from build123d import *

# Parameters (mm, degrees)
BOSS_EXTRUDE1_DEPTH = 3.175
CUT_EXTRUDE1_DEPTH  = 10
SKETCH3_R           = 2.0193
BOSS_EXTRUDE2_DEPTH = 3.175
FILLET1_R           = 10
FILLET2_R           = 50
SKETCH4_R           = 2.02
CUT_EXTRUDE2_DEPTH  = 10
SKETCH5_R           = 2.0193
BOSS_EXTRUDE3_DEPTH = 3.175
SKETCH6_W           = 3.175
SKETCH6_H           = 346.1216
CUT_EXTRUDE3_DEPTH  = 131.549169731


with BuildPart() as part:
    # Sketch1 → Boss-Extrude1 (new body)
    with BuildSketch(Plane.XY):
        Polygon((165.934536959, -16.66935), (157.315236959, -8.05005), (115.359952094, -8.05005), (89.959952094, -8.05005), (48.004667228, -8.05005), (39.385367228, -16.66935), (39.385367228, -40.05005), (39.385367228, -52.41105), (165.934536959, -56.67505), (165.934536959, -42.05005), align=None)
        with BuildLine():
            ThreePointArc((47.685367228, -44.38075), (49.704667228, -46.40005), (47.685367228, -48.41935))
            ThreePointArc((47.685367228, -48.41935), (45.666067228, -46.40005), (47.685367228, -44.38075))
        make_face(mode=Mode.SUBTRACT)
        with BuildLine():
            ThreePointArc((47.685367228, -12.63075), (49.704667228, -14.65005), (47.685367228, -16.66935))
            ThreePointArc((47.685367228, -16.66935), (45.666067228, -14.65005), (47.685367228, -12.63075))
        make_face(mode=Mode.SUBTRACT)
        with BuildLine():
            ThreePointArc((73.085367228, -44.38075), (75.104667228, -46.40005), (73.085367228, -48.41935))
            ThreePointArc((73.085367228, -48.41935), (71.066067228, -46.40005), (73.085367228, -44.38075))
        make_face(mode=Mode.SUBTRACT)
        with BuildLine():
            ThreePointArc((73.085367228, -12.63075), (75.104667228, -14.65005), (73.085367228, -16.66935))
            ThreePointArc((73.085367228, -16.66935), (71.066067228, -14.65005), (73.085367228, -12.63075))
        make_face(mode=Mode.SUBTRACT)
        with BuildLine():
            ThreePointArc((132.234536959, -44.38075), (134.253836959, -46.40005), (132.234536959, -48.41935))
            ThreePointArc((132.234536959, -48.41935), (130.215236959, -46.40005), (132.234536959, -44.38075))
        make_face(mode=Mode.SUBTRACT)
        with BuildLine():
            ThreePointArc((132.234536959, -12.63075), (134.253836959, -14.65005), (132.234536959, -16.66935))
            ThreePointArc((132.234536959, -16.66935), (130.215236959, -14.65005), (132.234536959, -12.63075))
        make_face(mode=Mode.SUBTRACT)
        with BuildLine():
            ThreePointArc((157.634536959, -44.38075), (159.653836959, -46.40005), (157.634536959, -48.41935))
            ThreePointArc((157.634536959, -48.41935), (155.615236959, -46.40005), (157.634536959, -44.38075))
        make_face(mode=Mode.SUBTRACT)
        with BuildLine():
            ThreePointArc((157.634536959, -12.63075), (159.653836959, -14.65005), (157.634536959, -16.66935))
            ThreePointArc((157.634536959, -16.66935), (155.615236959, -14.65005), (157.634536959, -12.63075))
        make_face(mode=Mode.SUBTRACT)
        Polygon((115.359952094, -8.05005), (157.315236959, -8.05005), (115.359952094, 33.905234866), align=None)
        Polygon((89.959952094, -8.05005), (115.359952094, -8.05005), (115.359952094, 33.905234866), (115.359952094, 203.394265134), (115.359952094, 245.34955), (89.959952094, 245.34955), (89.959952094, 203.394265134), (89.959952094, 33.905234866), align=None)
        Polygon((48.004667228, -8.05005), (89.959952094, -8.05005), (89.959952094, 33.905234866), align=None)
        Polygon((89.959952094, 245.34955), (115.359952094, 245.34955), (157.315236959, 245.34955), (165.934536959, 253.96885), (165.934536959, 279.34955), (165.934536959, 293.97455), (39.385367228, 289.71055), (39.385367228, 277.34955), (39.385367228, 253.96885), (48.004667228, 245.34955), align=None)
        with BuildLine():
            ThreePointArc((47.685367228, 253.96885), (49.704667228, 251.94955), (47.685367228, 249.93025))
            ThreePointArc((47.685367228, 249.93025), (45.666067228, 251.94955), (47.685367228, 253.96885))
        make_face(mode=Mode.SUBTRACT)
        with BuildLine():
            ThreePointArc((47.685367228, 285.71885), (49.704667228, 283.69955), (47.685367228, 281.68025))
            ThreePointArc((47.685367228, 281.68025), (45.666067228, 283.69955), (47.685367228, 285.71885))
        make_face(mode=Mode.SUBTRACT)
        with BuildLine():
            ThreePointArc((73.085367228, 253.96885), (75.104667228, 251.94955), (73.085367228, 249.93025))
            ThreePointArc((73.085367228, 249.93025), (71.066067228, 251.94955), (73.085367228, 253.96885))
        make_face(mode=Mode.SUBTRACT)
        with BuildLine():
            ThreePointArc((73.085367228, 285.71885), (75.104667228, 283.69955), (73.085367228, 281.68025))
            ThreePointArc((73.085367228, 281.68025), (71.066067228, 283.69955), (73.085367228, 285.71885))
        make_face(mode=Mode.SUBTRACT)
        with BuildLine():
            ThreePointArc((132.234536959, 253.96885), (134.253836959, 251.94955), (132.234536959, 249.93025))
            ThreePointArc((132.234536959, 249.93025), (130.215236959, 251.94955), (132.234536959, 253.96885))
        make_face(mode=Mode.SUBTRACT)
        with BuildLine():
            ThreePointArc((157.634536959, 253.96885), (159.653836959, 251.94955), (157.634536959, 249.93025))
            ThreePointArc((157.634536959, 249.93025), (155.615236959, 251.94955), (157.634536959, 253.96885))
        make_face(mode=Mode.SUBTRACT)
        with BuildLine():
            ThreePointArc((157.634536959, 285.71885), (159.653836959, 283.69955), (157.634536959, 281.68025))
            ThreePointArc((157.634536959, 281.68025), (155.615236959, 283.69955), (157.634536959, 285.71885))
        make_face(mode=Mode.SUBTRACT)
        Polygon((115.359952094, 245.34955), (115.359952094, 203.394265134), (157.315236959, 245.34955), align=None)
        Polygon((48.004667228, 245.34955), (89.959952094, 203.394265134), (89.959952094, 245.34955), align=None)
    extrude(amount=BOSS_EXTRUDE1_DEPTH)

    # Sketch2 → Cut-Extrude1 (cut)
    with BuildSketch(Plane.XY.offset(3.175)):
        Polygon((84.385367228, -52.41105), (39.385367228, -52.41105), (165.934536959, -56.67505), (165.934536959, -52.41105), (120.934536959, -52.41105), align=None)
        Polygon((120.934536959, 289.71055), (165.934536959, 289.71055), (165.934536959, 293.97455), (39.385367228, 289.71055), (84.385367228, 289.71055), align=None)
    extrude(amount=-CUT_EXTRUDE1_DEPTH, mode=Mode.SUBTRACT)

    # Sketch3 → Boss-Extrude2 (add)
    with BuildSketch(Plane.XY.offset(3.175)):
        Polygon((37.385367228, -15.840922875), (37.385367228, -54.41105), (167.934536959, -54.41105), (167.934536959, -15.840922875), (117.359952094, 34.73366199), (117.359952094, 202.56583801), (167.934536959, 253.140422875), (167.934536959, 291.71055), (37.385367228, 291.71055), (37.385367228, 253.140422875), (87.959952094, 202.56583801), (87.959952094, 34.73366199), align=None)
        with Locations((132.234536959, -46.40005)):
            Circle(SKETCH3_R, mode=Mode.SUBTRACT)
        with Locations((132.234536959, -14.65005)):
            Circle(SKETCH3_R, mode=Mode.SUBTRACT)
        with Locations((47.685367228, -14.65005)):
            Circle(SKETCH3_R, mode=Mode.SUBTRACT)
        with Locations((47.685367228, -46.40005)):
            Circle(SKETCH3_R, mode=Mode.SUBTRACT)
        with Locations((73.085367228, -46.40005)):
            Circle(SKETCH3_R, mode=Mode.SUBTRACT)
        with Locations((73.085367228, -14.65005)):
            Circle(SKETCH3_R, mode=Mode.SUBTRACT)
        with Locations((157.634536959, -14.65005)):
            Circle(SKETCH3_R, mode=Mode.SUBTRACT)
        with Locations((157.634536959, -46.40005)):
            Circle(SKETCH3_R, mode=Mode.SUBTRACT)
        with Locations((132.234536959, 251.94955)):
            Circle(SKETCH3_R, mode=Mode.SUBTRACT)
        with Locations((73.085367228, 251.94955)):
            Circle(SKETCH3_R, mode=Mode.SUBTRACT)
        with Locations((157.634536959, 251.94955)):
            Circle(SKETCH3_R, mode=Mode.SUBTRACT)
        with Locations((47.685367228, 251.94955)):
            Circle(SKETCH3_R, mode=Mode.SUBTRACT)
        with Locations((47.685367228, 283.69955)):
            Circle(SKETCH3_R, mode=Mode.SUBTRACT)
        with Locations((73.085367228, 283.69955)):
            Circle(SKETCH3_R, mode=Mode.SUBTRACT)
        with Locations((157.634536959, 283.69955)):
            Circle(SKETCH3_R, mode=Mode.SUBTRACT)
    extrude(amount=-BOSS_EXTRUDE2_DEPTH)

    # Fillet1
    fillet1_edges = [part.edges().sort_by_distance(p)[0] for p in [
        (37.385367228, -54.41105, 1.5875),
        (167.934536959, -54.41105, 1.5875),
        (167.934536959, -15.840922875, 1.5875),
        (167.934536959, 253.140422875, 1.5875),
        (167.934536959, 291.71055, 1.5875),
        (37.385367228, 291.71055, 1.5875),
        (37.385367228, 253.140422875, 1.5875),
        (37.385367228, -15.840922875, 1.5875),
    ]]
    fillet(fillet1_edges, radius=FILLET1_R)

    # Fillet2
    fillet2_edges = [part.edges().sort_by_distance(p)[0] for p in [
        (117.359952094, 34.73366199, 1.5875),
        (117.359952094, 202.56583801, 1.5875),
        (87.959952094, 202.56583801, 1.5875),
        (87.959952094, 34.73366199, 1.5875),
    ]]
    fillet(fillet2_edges, radius=FILLET2_R)

    # Sketch4 → Cut-Extrude2 (cut)
    with BuildSketch(Plane.XY.offset(3.175)):
        with Locations((132.234536959, 283.69955)):
            Circle(SKETCH4_R)
    extrude(amount=-CUT_EXTRUDE2_DEPTH, mode=Mode.SUBTRACT)

    # Sketch5 → Boss-Extrude3 (add)
    with BuildSketch(Plane.XY.offset(3.175)):
        with BuildLine():
            Line((167.934536959, -44.41105), (167.934536959, -16.63905))
            ThreePointArc((167.934536959, -16.63905), (165.005604771, -9.567982188), (157.934536959, -6.63905))
            Line((157.934536959, -6.63905), (47.385367228, -6.63905))
            ThreePointArc((47.385367228, -6.63905), (40.314299416, -9.567982188), (37.385367228, -16.63905))
            Line((37.385367228, -16.63905), (37.385367228, -44.41105))
            ThreePointArc((37.385367228, -44.41105), (40.314299416, -51.482117812), (47.385367228, -54.41105))
            Line((47.385367228, -54.41105), (157.934536959, -54.41105))
            ThreePointArc((157.934536959, -54.41105), (165.005604771, -51.482117812), (167.934536959, -44.41105))
        make_face()
        with Locations((47.685367228, -46.40005)):
            Circle(SKETCH5_R, mode=Mode.SUBTRACT)
        with Locations((73.085367228, -46.40005)):
            Circle(SKETCH5_R, mode=Mode.SUBTRACT)
        with Locations((132.234536959, -46.40005)):
            Circle(SKETCH5_R, mode=Mode.SUBTRACT)
        with Locations((157.634536959, -46.40005)):
            Circle(SKETCH5_R, mode=Mode.SUBTRACT)
        with Locations((47.685367228, -14.65005)):
            Circle(SKETCH5_R, mode=Mode.SUBTRACT)
        with Locations((73.085367228, -14.65005)):
            Circle(SKETCH5_R, mode=Mode.SUBTRACT)
        with Locations((132.234536959, -14.65005)):
            Circle(SKETCH5_R, mode=Mode.SUBTRACT)
        with Locations((157.634536959, -14.65005)):
            Circle(SKETCH5_R, mode=Mode.SUBTRACT)
    extrude(amount=BOSS_EXTRUDE3_DEPTH)

    # Sketch6 → Cut-Extrude3 (cut, through all)
    with BuildSketch(Plane.ZY.offset(-37.385367228)):
        with Locations((1.5875, 118.64975)):
            Rectangle(SKETCH6_W, SKETCH6_H)
    extrude(amount=-CUT_EXTRUDE3_DEPTH, mode=Mode.SUBTRACT)


solid = part.part
Here's how the part is built. I have some questions about the finished solid (model axes, mm). Round coordinates to 2 decimals unless told otherwise and drop trailing zeros. Order: outer loops, then holes, each group sorted by start corner. A loop starts at its lowest first (then second) coordinate and runs counter-clockwise, first axis right, second up. Notation, with made-up numbers: M -15.5,52 L 16.5,52 A12 ccw 16.5,67 Z; hole C -11,84.25 d3. An arc over 180 degrees is marked long. One line per question, with ' | ' between items.
1) I need wall thicknesses on line 1 (X direction, y = -46, z = 5.6); line 2 (X direction, y = -14, z = 5.35); line 3 (Y direction, x = 156, z = 3.9). Which ranges of each line are inside material? Lowest first, please.
Checked values:
line 1: x = 37.51 to 45.71, 49.66 to 71.11, 75.06 to 130.26, 134.21 to 155.66, 159.61 to 167.81 | line 2: x = 37.74 to 45.77, 49.6 to 71.17, 75 to 130.32, 134.15 to 155.72, 159.55 to 167.58 | line 3: y = -54.41 to -47.59, -45.21 to -15.84, -13.46 to -6.64
2) I'm going to push a flat-ended pin straight in: pin 1 Ø4.5 at (x, y) = (73.09, -14.65) entering from +Z. Where does the tip first touch, or does it pass through?
Checked values:
pin 1: stops at z = 6.35
3) Imagine slicing it at C-C, the plane y = -51. Write out the boundary of the cut face in (x, z) (3 decimals), plus the area to 3 significant figures.
Checked values:
outline: M 39.863,3.175 L 165.457,3.175 L 165.457,6.35 L 39.863,6.35 Z | area: 399 mm²
4) We'd pull the mould along X, two halves only. Please class faces 1 (the cylindrical face through (40.392, -9.491, 4.74)), 2 (the cylindrical face through (71.07, -14.56, 4.74)), 3 (the flat face through (102, -31, 3.175)): released by +X, released by -X, zero draft, split by the parting line, or undercut.
Checked values:
face 1: released by -X | face 2: undercut | face 3: zero draft
5) Imagine slicing it at A-A, the plane x = 131.5. Write out the boundary of the cut face in (y, z) (3 decimals).
Checked values:
outline: M -54.411,3.175 L -48.281,3.175 L -48.281,6.35 L -54.411,6.35 Z; M -44.519,3.175 L -16.531,3.175 L -16.531,6.35 L -44.519,6.35 Z; M -12.769,3.175 L -6.639,3.175 L -6.639,6.35 L -12.769,6.35 Z
